Work out the finished part from the listing and answer in its coordinate system (mm). A direction names the side the tool comes from. Give positions to 0.01 mm unless a question says otherwise; leave off trailing zeros. Write each loop counter-clockwise with the first axis right and the second up, starting at its lowest first coordinate (ties: lowest second). Pieces come first, ordered by that corner, then holes.
1) Determine the mould class of faces 4 (the face through (72.8, 23.27, -32.86)), 5 (the face through (40, 0, -39)), 6 (the face through (39, 23, -20)), 7 (the face through (78, 17, -20)) for opening direction X: pulls with the +X half, pulls with the -X half, needs draft (parallel to the pull), parting line crosses it, or undercut.
2) Find section B-B (x = 52.5). Determine the outline of the cut face in (y, z), plus the area to 3 significant figures.
3) Find section A-A (y = 15.5). Determine the outline of the cut face in (x, z), plus the area to 3 significant figures.
4) Find section C-C (y = 22.25). Count the separate pieces of the cut face and the enclosed holes in it, plus the area to 3 significant figures.
5) Straight lines are drawn through the part: probe 1 along X at (y, z) = (8.5, -35.8); probe 2 along X at (y, z) = (24.7, -20); probe 3 along X at (y, z) = (24.7, -15). For each, find the intervals that lie inside material, in ascending order.
6) Find section D-D (z = -15). Determine the outline of the cut face in (x, y).
7) A tool of negligible diameter and unlimited length cuts with its end or side. For faces 1 (the face through (60, 18, -8)), 2 (the face through (40, 22, -34)), 3 (the face through (78, 23, -8.4)), from which of +Z, -Z, +X, -X, +Y, -Y can it reach the whole face along a straight path? Write none if from no direction.
8) Given pin 1 Ø3 at (x, z) = (71, -19) entering from -Y; pin 2 Ø6 at (x, z) = (21.5, -19) entering from -Y; pin 3 Ø4 at (x, z) = (51, -22.5) entering from -Y, each flat-ended and moving along its own axis, determine where each tip first touches the part or whether it passes through.
```python
from build123d import *

# Parameters (mm, degrees)
ESQUISSE1_W              = 80
ESQUISSE1_H              = 40
BOSS_EXTRU_1_DEPTH       = 25
ENL_V_MAT_EXTRU_4_DEPTH  = 78
ESQUISSE6_W              = 2
ESQUISSE6_H              = 25
BOSS_EXTRU_3_DEPTH       = 40
ESQUISSE7_R              = 11
ENL_V_MAT_EXTRU_5_DEPTH  = 93.870878105
ESQUISSE8_W              = 60
ESQUISSE8_H              = 36
ENL_V_MAT_EXTRU_6_DEPTH  = 23
ESQUISSE9_W              = 10
ESQUISSE9_H              = 9
BOSS_EXTRU_4_DEPTH       = 23
ESQUISSE10_R             = 2.1
ENL_V_MAT_EXTRU_8_DEPTH  = 93.870878105
ESQUISSE11_R             = 2.75
ENL_V_MAT_EXTRU_9_DEPTH  = 93.870878105
CHANFREIN1_SIZE          = 1
ESQUISSE12_R             = 4.2
ESQUISSE12_R_2           = 2.1
ENL_V_MAT_EXTRU_10_DEPTH = 3.5
CONG_1_R                 = 4.2
ESQUISSE13_W             = 7
ESQUISSE13_H             = 7
BOSS_EXTRU_5_DEPTH       = 3
ESQUISSE14_W             = 20
ESQUISSE14_H             = 2
BOSS_EXTRU_16_DEPTH      = 5
ESQUISSE15_W             = 20
ESQUISSE15_H             = 2
BOSS_EXTRU_17_DEPTH      = 7
ESQUISSE17_W             = 20
ESQUISSE17_H             = 2
BOSS_EXTRU_18_DEPTH      = 11
ESQUISSE18_R             = 1.5
BOSS_EXTRU_19_DEPTH      = 3


with BuildPart() as part:
    # Esquisse1 → Boss.-Extru.1 (new body)
    with BuildSketch(Plane(origin=(0, 0, 0), x_dir=(1, 0, 0), z_dir=(0, 1, 0))):
        with Locations((40, 20)):
            Rectangle(ESQUISSE1_W, ESQUISSE1_H)
    extrude(amount=BOSS_EXTRU_1_DEPTH)

    # Esquisse5 → Enlèv. mat.-Extru.4 (cut)
    with BuildSketch(Plane.ZY):
        with BuildLine():
            Line((-2, 23), (-38, 23))
            Line((-38, 23), (-38, 2))
            Line((-38, 2), (-32.845232579, 2))
            ThreePointArc((-32.845232579, 2), (-20, 13), (-7.154767421, 2))
            Line((-7.154767421, 2), (-2, 2))
            Line((-2, 2), (-2, 23))
        make_face()
    extrude(amount=-ENL_V_MAT_EXTRU_4_DEPTH, mode=Mode.SUBTRACT)

    # Esquisse6 → Boss.-Extru.3 (add)
    with BuildSketch(Plane(origin=(0, 0, -40), x_dir=(-1, 0, 0), z_dir=(0, 0, -1))):
        with Locations((-1, 12.5)):
            Rectangle(ESQUISSE6_W, ESQUISSE6_H)
    extrude(amount=-BOSS_EXTRU_3_DEPTH)

    # Esquisse7 → Enlèv. mat.-Extru.5 (cut, through all)
    with BuildSketch(Plane.ZY):
        with Locations((-20, 0)):
            Circle(ESQUISSE7_R)
    extrude(amount=-ENL_V_MAT_EXTRU_5_DEPTH, mode=Mode.SUBTRACT)

    # Esquisse8 → Enlèv. mat.-Extru.6 (cut)
    with BuildSketch(Plane.XZ):
        with Locations((40, -20)):
            Rectangle(ESQUISSE8_W, ESQUISSE8_H)
    extrude(amount=-ENL_V_MAT_EXTRU_6_DEPTH, mode=Mode.SUBTRACT)

    # Esquisse9 → Boss.-Extru.4 (add)
    with BuildSketch(Plane(origin=(0, 25, 0), x_dir=(1, 0, 0), z_dir=(0, 1, 0))):
        with Locations((75, 4.5)):
            Rectangle(ESQUISSE9_W, ESQUISSE9_H)
        with Locations((5, 4.5)):
            Rectangle(ESQUISSE9_W, ESQUISSE9_H)
        with Locations((5, 35.5)):
            Rectangle(ESQUISSE9_W, ESQUISSE9_H)
        with Locations((75, 35.5)):
            Rectangle(ESQUISSE9_W, ESQUISSE9_H)
    extrude(amount=-BOSS_EXTRU_4_DEPTH)

    # Esquisse10 → Enlèv. mat.-Extru.8 (cut, through all)
    with BuildSketch(Plane(origin=(0, 25, 0), x_dir=(1, 0, 0), z_dir=(0, 1, 0))):
        with Locations(Location((75.8, 35.8, 0), (0, 0, 270))):
            Circle(ESQUISSE10_R)
        with Locations(Location((75.8, 4.2, 0), (0, 0, 270))):
            Circle(ESQUISSE10_R)
        with Locations(Location((4.2, 4.2, 0), (0, 0, 270))):
            Circle(ESQUISSE10_R)
        with Locations(Location((4.2, 35.8, 0), (0, 0, 270))):
            Circle(ESQUISSE10_R)
    extrude(amount=-ENL_V_MAT_EXTRU_8_DEPTH, mode=Mode.SUBTRACT)

    # Esquisse11 → Enlèv. mat.-Extru.9 (cut, through all)
    with BuildSketch(Plane(origin=(0, 25, 0), x_dir=(1, 0, 0), z_dir=(0, 1, 0))):
        with Locations(Location((60, 20, 0), (0, 0, 270))):
            Circle(ESQUISSE11_R)
        with Locations(Location((40, 15, 0), (0, 0, 270))):
            Circle(ESQUISSE11_R)
        with Locations(Location((20, 20, 0), (0, 0, 270))):
            Circle(ESQUISSE11_R)
    extrude(amount=-ENL_V_MAT_EXTRU_9_DEPTH, mode=Mode.SUBTRACT)

    # Chanfrein1
    chanfrein1_edges = [part.edges().sort_by_distance(p)[0] for p in [
        (60, 23, -22.75),
        (40, 23, -17.75),
        (20, 23, -22.75),
    ]]
    chamfer(chanfrein1_edges, length=CHANFREIN1_SIZE)

    # Esquisse12 → Enlèv. mat.-Extru.10 (cut)
    with BuildSketch(Plane(origin=(0, 25, 0), x_dir=(1, 0, 0), z_dir=(0, 1, 0))):
        with BuildLine():
            Line((71.6, 4.2), (71.6, 0))
            Line((71.6, 0), (75.8, 0))
            ThreePointArc((75.8, 0), (72.830151519, 1.230151519), (71.6, 4.2))
        make_face()
        with Locations((75.8, 4.2)):
            Circle(ESQUISSE12_R)
        with Locations(Location((75.8, 4.2, 0), (0, 0, 270))):
            Circle(ESQUISSE12_R_2, mode=Mode.SUBTRACT)
        with BuildLine():
            ThreePointArc((80, 4.2), (78.769848481, 1.230151519), (75.8, 0))
            Line((75.8, 0), (80, 0))
            Line((80, 0), (80, 4.2))
        make_face()
        with BuildLine():
            Line((80, 8.4), (75.8, 8.4))
            ThreePointArc((75.8, 8.4), (78.769848481, 7.169848481), (80, 4.2))
            Line((80, 4.2), (80, 8.4))
        make_face()
        with BuildLine():
            Line((75.8, 31.6), (80, 31.6))
            Line((80, 31.6), (80, 35.8))
            ThreePointArc((80, 35.8), (78.769848481, 32.830151519), (75.8, 31.6))
        make_face()
        with Locations((75.8, 35.8)):
            Circle(ESQUISSE12_R)
        with Locations(Location((75.8, 35.8, 0), (0, 0, 270))):
            Circle(ESQUISSE12_R_2, mode=Mode.SUBTRACT)
        with BuildLine():
            ThreePointArc((75.8, 40), (78.769848481, 38.769848481), (80, 35.8))
            Line((80, 35.8), (80, 40))
            Line((80, 40), (75.8, 40))
        make_face()
        with BuildLine():
            Line((71.6, 40), (71.6, 35.8))
            ThreePointArc((71.6, 35.8), (72.830151519, 38.769848481), (75.8, 40))
            Line((75.8, 40), (71.6, 40))
        make_face()
        with BuildLine():
            Line((0, 35.8), (0, 31.6))
            Line((0, 31.6), (4.2, 31.6))
            ThreePointArc((4.2, 31.6), (1.230151519, 32.830151519), (0, 35.8))
        make_face()
        with Locations((4.2, 35.8)):
            Circle(ESQUISSE12_R)
        with Locations(Location((4.2, 35.8, 0), (0, 0, 270))):
            Circle(ESQUISSE12_R_2, mode=Mode.SUBTRACT)
        with BuildLine():
            Line((0, 40), (0, 35.8))
            ThreePointArc((0, 35.8), (1.230151526, 38.769848488), (4.200000019, 40))
            Line((4.200000019, 40), (0, 40))
        make_face()
        with BuildLine():
            ThreePointArc((4.200000019, 40), (7.169848488, 38.769848474), (8.4, 35.8))
            Line((8.4, 35.8), (8.4, 40))
            Line((8.4, 40), (4.200000019, 40))
        make_face()
        with BuildLine():
            ThreePointArc((0, 4.200000008), (1.230151522, 7.169848484), (4.2, 8.4))
            Line((4.2, 8.4), (0, 8.4))
            Line((0, 8.4), (0, 4.200000008))
        make_face()
        with Locations((4.2, 4.2)):
            Circle(ESQUISSE12_R)
        with Locations(Location((4.2, 4.2, 0), (0, 0, 270))):
            Circle(ESQUISSE12_R_2, mode=Mode.SUBTRACT)
        with BuildLine():
            Line((0, 0), (4.2, 0))
            ThreePointArc((4.2, 0), (1.230151516, 1.230151522), (0, 4.200000008))
            Line((0, 4.200000008), (0, 0))
        make_face()
        with BuildLine():
            Line((4.2, 0), (8.4, 0))
            Line((8.4, 0), (8.4, 4.2))
            ThreePointArc((8.4, 4.2), (7.169848481, 1.230151519), (4.2, 0))
        make_face()
    extrude(amount=-ENL_V_MAT_EXTRU_10_DEPTH, mode=Mode.SUBTRACT)

    # Congé1
    cong_1_edges = [part.edges().sort_by_distance(p)[0] for p in [
        (80, 10.75, 0),
        (80, 10.75, -40),
        (0, 10.75, -40),
        (0, 10.75, 0),
    ]]
    fillet(cong_1_edges, radius=CONG_1_R)

    # Esquisse13 → Boss.-Extru.5 (add)
    with BuildSketch(Plane.XZ.offset(-23)):
        with BuildLine():
            Line((32.45, -21), (47.55, -21))
            ThreePointArc((47.55, -21), (50.55, -24), (47.55, -27))
            Line((47.55, -27), (32.45, -27))
            ThreePointArc((32.45, -27), (29.45, -24), (32.45, -21))
        make_face()
        with Locations((40, -30.5)):
            Rectangle(ESQUISSE13_W, ESQUISSE13_H)
    extrude(amount=BOSS_EXTRU_5_DEPTH)

    # Esquisse14 → Boss.-Extru.16 (add)
    with BuildSketch(Plane.XZ.offset(-23)):
        with Locations((60, -8)):
            Rectangle(ESQUISSE14_W, ESQUISSE14_H)
    extrude(amount=BOSS_EXTRU_16_DEPTH)

    # Esquisse15 → Boss.-Extru.17 (add)
    with BuildSketch(Plane(origin=(0, 0, -2), x_dir=(-1, 0, 0), z_dir=(0, 0, -1))):
        with Locations((-60, 1)):
            Rectangle(ESQUISSE15_W, ESQUISSE15_H)
    extrude(amount=BOSS_EXTRU_17_DEPTH)

    # Esquisse17 → Boss.-Extru.18 (add)
    with BuildSketch(Plane.XZ):
        with Locations((60, -8)):
            Rectangle(ESQUISSE17_W, ESQUISSE17_H)
    extrude(amount=-BOSS_EXTRU_18_DEPTH)

    # Esquisse18 → Boss.-Extru.19 (add)
    with BuildSketch(Plane.XZ.offset(-20)):
        with Locations(Location((32.45, -24, 0), (0, 0, 270))):
            Circle(ESQUISSE18_R)
        with Locations(Location((47.55, -24, 0), (0, 0, 270))):
            Circle(ESQUISSE18_R)
    extrude(amount=BOSS_EXTRU_19_DEPTH)


solid = part.part
```
Results:
1. face 4: pulls with the +X half
1. face 5: needs draft
1. face 6: undercut
1. face 7: undercut
2. outline: (0, -40) - (25, -40) - (25, 0) - (0, 0) - (0, -9) - (11, -9) - (11, -7) - (2, -7) - (2, -2) - (23, -2) - (23, -7) - (18, -7) - (18, -9) - (23, -9) - (23, -38) - (0, -38) - close
2. area: 214 mm2
3. outline: (0, -35.8) arc R4.2 ccw to (4.2, -40) - (75.8, -40) arc R4.2 ccw to (80, -35.8) - (80, -4.2) arc R4.2 ccw to (75.8, 0) - (4.2, 0) arc R4.2 ccw to (0, -4.2) - close; hole (2, -31) - (10, -31) - (10, -38) - (70, -38) - (70, -31) - (78, -31) - (78, -9) - (70, -9) - (70, -2) - (10, -2) - (10, -9) - (2, -9) - close; hole circle Ø4.2 at (4.2, -35.8); hole circle Ø4.2 at (4.2, -4.2); hole circle Ø4.2 at (75.8, -35.8); hole circle Ø4.2 at (75.8, -4.2)
3. area: 617 mm2
4. separate pieces: 2
4. enclosed holes: 1
4. area: 629 mm2
5. probe 1: x = 0 to 2.1, 6.3 to 10, 70 to 73.7, 77.9 to 80
5. probe 2: x = 0 to 17.25, 22.75 to 57.25, 62.75 to 80
5. probe 3: x = 0 to 37.25, 42.75 to 80
6. outline: (0, 9.8) - (10, 9.8) - (10, 12) - (2, 12) - (2, 23) - (36.25, 23) - (37.25, 24) - (37.25, 25) - (0, 25) - close; (42.75, 24) - (43.75, 23) - (78, 23) - (78, 12) - (70, 12) - (70, 9.8) - (80, 9.8) - (80, 25) - (42.75, 25) - close
7. face 1: none
7. face 2: -Y
7. face 3: +Z, +X, +Y
8. pin 1: stops at y = 10.71
8. pin 2: stops at y = 23
8. pin 3: stops at y = 20
